Can you work these out from the model? Positions are in its coordinate system, mm. A direction names the side the tool comes from. Give positions to 0.01 mm unless a question says otherwise; leave off trailing zeros. Write each loop counter-clockwise with the first axis right and the second up, starting at its lowest first coordinate (ties: lowest second). Pieces come first, ordered by that corner, then holes.
from build123d import *

# Parameters (mm, degrees)
SKETCH1_W           = 8.6
SKETCH1_H           = 27
BOSS_EXTRUDE1_DEPTH = 31.5
SKETCH2_W           = 27
SKETCH2_H           = 3
BOSS_EXTRUDE2_DEPTH = 40.5
SKETCH3_W           = 3
SKETCH3_H           = 28.5
BOSS_EXTRUDE3_DEPTH = 40.5
SKETCH4_W           = 8.6
SKETCH4_H           = 27
BOSS_EXTRUDE4_DEPTH = 31.5
CUT_EXTRUDE8_DEPTH  = 10
FILLET1_R           = 3
SKETCH5_R           = 2.2
CUT_EXTRUDE1_DEPTH  = 5
SKETCH6_W           = 17.5
SKETCH6_H           = 10
CUT_EXTRUDE2_DEPTH  = 10
FILLET3_R           = 1
SKETCH9_W           = 27
SKETCH9_H           = 5
BOSS_EXTRUDE5_DEPTH = 22.5
SKETCH10_R          = 2.2
CUT_EXTRUDE5_DEPTH  = 100
FILLET4_R           = 3
FILLET5_R           = 0.3
SKETCH12_W          = 14.05
SKETCH12_H          = 27
CUT_EXTRUDE6_DEPTH  = 10
FILLET6_R           = 3


with BuildPart() as part:
    # Sketch1 → Boss-Extrude1 (new body)
    with BuildSketch(Plane(origin=(0, 0, 0), x_dir=(1, 0, 0), z_dir=(0, 1, 0))):
        with Locations((4.3, 0)):
            Rectangle(SKETCH1_W, SKETCH1_H)
    extrude(amount=BOSS_EXTRUDE1_DEPTH)

    # Sketch2 → Boss-Extrude2 (add)
    with BuildSketch(Plane(origin=(8.6, 0, 0), x_dir=(0, 0, -1), z_dir=(1, 0, 0))):
        with Locations((0, 1.5)):
            Rectangle(SKETCH2_W, SKETCH2_H)
    extrude(amount=BOSS_EXTRUDE2_DEPTH)

    # Sketch3 → Boss-Extrude3 (add)
    with BuildSketch(Plane(origin=(8.6, 0, 0), x_dir=(0, 0, -1), z_dir=(1, 0, 0))):
        with Locations((12, 17.25)):
            Rectangle(SKETCH3_W, SKETCH3_H)
    extrude(amount=BOSS_EXTRUDE3_DEPTH)

    # Sketch4 → Boss-Extrude4 (add)
    with BuildSketch(Plane(origin=(0, 31.5, 0), x_dir=(1, 0, 0), z_dir=(0, 1, 0))):
        with Locations((53.4, 0)):
            Rectangle(SKETCH4_W, SKETCH4_H)
    extrude(amount=-BOSS_EXTRUDE4_DEPTH)

    # Sketch15 → Cut-Extrude8 (cut)
    with BuildSketch(Plane.XY.offset(-10.5)):
        with BuildLine():
            Line((31.35, 8.25), (31.35, 26.25))
            ThreePointArc((31.35, 26.25), (28.85, 28.75), (26.35, 26.25))
            Line((26.35, 26.25), (26.35, 8.25))
            ThreePointArc((26.35, 8.25), (28.85, 5.75), (31.35, 8.25))
        make_face()
        with BuildLine():
            Line((42.725, 8.25), (42.725, 26.25))
            ThreePointArc((42.725, 26.25), (40.225, 28.75), (37.725, 26.25))
            Line((37.725, 26.25), (37.725, 8.25))
            ThreePointArc((37.725, 8.25), (40.225, 5.75), (42.725, 8.25))
        make_face()
        with BuildLine():
            Line((19.975, 8.25), (19.975, 26.25))
            ThreePointArc((19.975, 26.25), (17.475, 28.75), (14.975, 26.25))
            Line((14.975, 26.25), (14.975, 8.25))
            ThreePointArc((14.975, 8.25), (17.475, 5.75), (19.975, 8.25))
        make_face()
    extrude(amount=-CUT_EXTRUDE8_DEPTH, mode=Mode.SUBTRACT)

    # Fillet1
    fillet1_edges = [part.edges().sort_by_distance(p)[0] for p in [
        (57.7, 15.75, -13.5),
        (57.7, 15.75, 13.5),
        (49.1, 17.25, 13.5),
        (8.6, 17.25, 13.5),
    ]]
    fillet(fillet1_edges, radius=FILLET1_R)

    # Sketch5 → Cut-Extrude1 (cut)
    with BuildSketch(Plane(origin=(0, 31.5, 0), x_dir=(1, 0, 0), z_dir=(0, 1, 0))):
        with Locations(Location((53.4, 4.95, 0), (0, 0, 270))):
            Circle(SKETCH5_R)
        with Locations(Location((53.4, -4.95, 0), (0, 0, 270))):
            Circle(SKETCH5_R)
        with Locations(Location((4.3, 4.95, 0), (0, 0, 270))):
            Circle(SKETCH5_R)
        with Locations(Location((4.3, -4.95, 0), (0, 0, 270))):
            Circle(SKETCH5_R)
    extrude(amount=-CUT_EXTRUDE1_DEPTH, mode=Mode.SUBTRACT)

    # Sketch6 → Cut-Extrude2 (cut)
    with BuildSketch(Plane.ZY.offset(-49.1)):
        with Locations((4.75, 10)):
            Rectangle(SKETCH6_W, SKETCH6_H)
    extrude(amount=-CUT_EXTRUDE2_DEPTH, mode=Mode.SUBTRACT)

    # Fillet3
    fillet3_edges = [part.edges().sort_by_distance(p)[0] for p in [
        (56.821320344, 5, 12.621320344),
        (56.821320344, 15, 12.621320344),
        (57.7, 10, -4),
        (49.1, 5, 3.25),
        (49.1, 15, 3.25),
        (49.1, 10, -4),
        (49.978679656, 15, 12.621320344),
        (57.7, 15, 3.25),
        (53.4, 15, 13.5),
        (49.978679656, 5, 12.621320344),
        (57.7, 5, 3.25),
        (53.4, 15, -4),
        (53.4, 5, 13.5),
        (53.4, 5, -4),
    ]]
    fillet(fillet3_edges, radius=FILLET3_R)

    # Sketch9 → Boss-Extrude5 (add)
    with BuildSketch(Plane.ZY):
        with Locations((0, 29)):
            Rectangle(SKETCH9_W, SKETCH9_H)
        with Locations((0, 2.5)):
            Rectangle(SKETCH9_W, SKETCH9_H)
    extrude(amount=BOSS_EXTRUDE5_DEPTH)

    # Sketch10 → Cut-Extrude5 (cut)
    with BuildSketch(Plane(origin=(0, 31.5, 0), x_dir=(1, 0, 0), z_dir=(0, 1, 0))):
        with Locations(Location((-5.3, 4.95, 0), (0, 0, 90))):
            Circle(SKETCH10_R)
        with Locations(Location((-5.3, -4.95, 0), (0, 0, 90))):
            Circle(SKETCH10_R)
        with Locations(Location((-17.2, -4.95, 0), (0, 0, 90))):
            Circle(SKETCH10_R)
        with Locations(Location((-17.2, 4.95, 0), (0, 0, 90))):
            Circle(SKETCH10_R)
    extrude(amount=-CUT_EXTRUDE5_DEPTH, mode=Mode.SUBTRACT)

    # Fillet4
    fillet4_edges = [part.edges().sort_by_distance(p)[0] for p in [
        (0, 15.75, 13.5),
        (0, 15.75, -13.5),
        (-22.5, 2.5, 13.5),
        (-22.5, 2.5, -13.5),
    ]]
    fillet(fillet4_edges, radius=FILLET4_R)

    # Fillet5
    # the kernel refuses this fillet: 0.3 mm, written as the material it adds along each edge
    with BuildSketch(Plane(origin=(0, 5, 10.5), x_dir=(0, 1, 0), z_dir=(0, 0, -1))) as fillet5_piece_1:
        with BuildLine():
            CenterArc((FILLET5_R, -FILLET5_R), FILLET5_R, 90, 90)
            Line((0, -FILLET5_R), (0, 0))
            Line((0, 0), (FILLET5_R, 0))
        make_face()
    extrude(amount=21)
    with BuildSketch(Plane(origin=(0, 26.5, 10.5), x_dir=(0, -1, 0), z_dir=(0, 0, -1))) as fillet5_piece_2:
        with BuildLine():
            CenterArc((FILLET5_R, FILLET5_R), FILLET5_R, 180, 90)
            Line((0, FILLET5_R), (0, 0))
            Line((0, 0), (FILLET5_R, 0))
        make_face()
    extrude(amount=21)
    with BuildSketch(Plane(origin=(3, 5, -10.5), x_dir=(-1, 0, 0), z_dir=(0, 0, 1))) as fillet5_piece_3_section:
        with BuildLine():
            CenterArc((3 + FILLET5_R, -FILLET5_R), FILLET5_R, 90, 90)
            Line((3 + FILLET5_R, 0), (3, 0))
            Line((3, 0), (3, -FILLET5_R))
        make_face()
    fillet5_piece_3 = revolve(axis=Axis((3, 5, -10.5), (0, -1, 0)), revolution_arc=104.329698924, mode=Mode.PRIVATE)
    fillet5_piece_3 = split(fillet5_piece_3, bisect_by=Plane(origin=(0.81861369, 5.084946104, -13.5), z_dir=(0, 0, 1)), keep=Keep.TOP, mode=Mode.PRIVATE)
    add(fillet5_piece_3)
    with BuildSketch(Plane(origin=(3, 26.5, -10.5), x_dir=(-1, 0, 0), z_dir=(0, 0, 1))) as fillet5_piece_4_section:
        with BuildLine():
            CenterArc((3 + FILLET5_R, FILLET5_R), FILLET5_R, 180, 90)
            Line((3 + FILLET5_R, 0), (3, 0))
            Line((3, 0), (3, FILLET5_R))
        make_face()
    fillet5_piece_4 = revolve(axis=Axis((3, 26.5, -10.5), (0, -1, 0)), revolution_arc=104.329698924, mode=Mode.PRIVATE)
    fillet5_piece_4 = split(fillet5_piece_4, bisect_by=Plane(origin=(0.81861369, 26.415053896, -13.5), z_dir=(0, 0, 1)), keep=Keep.TOP, mode=Mode.PRIVATE)
    add(fillet5_piece_4)
    with BuildSketch(Plane(origin=(3, 5, 10.5), x_dir=(0.24750126301206385, 0, 0.968887570777659), z_dir=(0.968887570777659, 0, -0.24750126301206385))) as fillet5_piece_5_section:
        with BuildLine():
            CenterArc((3 + FILLET5_R, -FILLET5_R), FILLET5_R, 90, 90)
            Line((3 + FILLET5_R, 0), (3, 0))
            Line((3, 0), (3, -FILLET5_R))
        make_face()
    fillet5_piece_5 = revolve(axis=Axis((3, 5, 10.5), (0, -1, 0)), revolution_arc=104.329698924, mode=Mode.PRIVATE)
    fillet5_piece_5 = split(fillet5_piece_5, bisect_by=Plane(origin=(0.818613701, 5.084946089, 13.5), z_dir=(0, 0, -1)), keep=Keep.TOP, mode=Mode.PRIVATE)
    add(fillet5_piece_5)
    with BuildSketch(Plane(origin=(3, 26.5, 10.5), x_dir=(0.24750126301206454, 0, 0.9688875707776589), z_dir=(0.9688875707776589, 0, -0.24750126301206454))) as fillet5_piece_6_section:
        with BuildLine():
            CenterArc((3 + FILLET5_R, FILLET5_R), FILLET5_R, 180, 90)
            Line((3, FILLET5_R), (3, 0))
            Line((3, 0), (3 + FILLET5_R, 0))
        make_face()
    fillet5_piece_6 = revolve(axis=Axis((3, 26.5, 10.5), (0, -1, 0)), revolution_arc=104.329698924, mode=Mode.PRIVATE)
    fillet5_piece_6 = split(fillet5_piece_6, bisect_by=Plane(origin=(0.818613746, 26.41505391, 13.5), z_dir=(0, 0, -1)), keep=Keep.TOP, mode=Mode.PRIVATE)
    add(fillet5_piece_6)

    # Sketch12 → Cut-Extrude6 (cut)
    with BuildSketch(Plane(origin=(0, 31.5, 0), x_dir=(1, 0, 0), z_dir=(0, 1, 0))):
        with Locations((-15.475, 0)):
            Rectangle(SKETCH12_W, SKETCH12_H)
    extrude(amount=-CUT_EXTRUDE6_DEPTH, mode=Mode.SUBTRACT)

    # Fillet6
    fillet6_edges = [part.edges().sort_by_distance(p)[0] for p in [
        (-8.45, 29, -13.5),
        (-8.45, 29, 13.5),
    ]]
    fillet(fillet6_edges, radius=FILLET6_R)


solid = part.part
(1) If I drill on L1, parallel to Z at x = -17.2, y = 2.65; L2, parallel to X at y = 29.8, z = -4.95; L3, parallel to X at y = 1.75, z = 4.95, over which ranges is the centre line in solid material (lowest first)?
Returned:
L1: z = -13.5 to -7.15, -2.75 to 2.75, 7.15 to 13.5
L2: x = -8.45 to -7.5, -3.1 to 2.1, 6.5 to 8.6, 49.1 to 51.2, 55.6 to 57.7
L3: x = -22.5 to -19.4, -15 to -7.5, -3.1 to 57.7
(2) Imagine slicing it at D-D, the plane x = 4.3. Write out the boundary of the cut face in (y, z).
Returned:
outline: (0, -13.5) - (31.5, -13.5) - (31.5, -7.15) - (26.5, -7.15) - (26.5, -2.75) - (31.5, -2.75) - (31.5, 2.75) - (26.5, 2.75) - (26.5, 7.15) - (31.5, 7.15) - (31.5, 13.5) - (0, 13.5) - close
(3) Imagine slicing it at C-C, the plane x = -17.2. Write out the boundary of the cut face in (y, z).
Returned:
outline: (0, -13.5) - (5, -13.5) - (5, -7.15) - (0, -7.15) - close; (0, -2.75) - (5, -2.75) - (5, 2.75) - (0, 2.75) - close; (0, 7.15) - (5, 7.15) - (5, 13.5) - (0, 13.5) - close
(4) Imagine slicing it at A-A, the plane z = -1.75. Write out the boundary of the cut face in (x, y).
Returned:
outline: (-22.5, 0) - (57.7, 0) - (57.7, 4) arc R1 ccw to (56.7, 5) - (50.1, 5) arc R1 ccw to (49.1, 4) - (49.1, 3) - (8.6, 3) - (8.6, 31.5) - (-8.45, 31.5) - (-8.45, 26.5) - (-0.3, 26.5) arc R0.3 cw to (0, 26.2) - (0, 5.3) arc R0.3 cw to (-0.3, 5) - (-22.5, 5) - close; (49.1, 16) arc R1 ccw to (50.1, 15) - (56.7, 15) arc R1 ccw to (57.7, 16) - (57.7, 31.5) - (49.1, 31.5) - close
(5) Will these pins go through, and if not, where does the flat tip stop? P1, Ø0.9, axis at y = 17.5, z = -12.5, coming from the +X side; P2, Ø1, axis at x = 4, z = 5, coming from the +Y side; P3, Ø5.5, axis at x = 52.5, y = 12, coming from the +Z side.
Returned:
P1: stops at x = 57.27
P2: stops at y = 26.5
P3: stops at z = -3.66
(6) If we mould it in two halves opening along Z, with no side actions, what happens to faces 1 (the face through (0.86, 15.9, 12.6)), 2 (the face through (4, 26.5, 5)), 3 (the face through (49.1, 21, -2)), 4 (the face through (5.79, 29.04, -6.57))? For each: +Z half, -Z half, draft (parallel to the pull), parting line (faces both ways), or undercut.
Returned:
face 1: +Z half
face 2: undercut
face 3: draft
face 4: undercut
(7) Imagine slicing it at B-B, the plane y = 22.5. Write out the boundary of the cut face in (x, z) (3 decimals), plus the area to 3 significant figures.
Returned:
outline: (0, -10.5) arc R3 ccw to (3, -13.5) - (14.975, -13.5) - (14.975, -10.5) - (8.6, -10.5) - (8.6, 10.5) arc R3 ccw to (5.6, 13.5) - (3, 13.5) arc R3 ccw to (0, 10.5) - close; (19.975, -13.5) - (26.35, -13.5) - (26.35, -10.5) - (19.975, -10.5) - close; (31.35, -13.5) - (37.725, -13.5) - (37.725, -10.5) - (31.35, -10.5) - close; (42.725, -13.5) - (54.7, -13.5) arc R3 ccw to (57.7, -10.5) - (57.7, 10.5) arc R3 ccw to (54.7, 13.5) - (52.1, 13.5) arc R3 ccw to (49.1, 10.5) - (49.1, -10.5) - (42.725, -10.5) - close
area: 529 mm2
(8) For faces 5 (the face through (0.9, 15.9, -12.64)), 6 (the face through (53, 26.5, -5)), 7 (the face through (31.35, 17, -12)), 8 (the face through (-6.79, 29.04, 6.57)), 9 (the face through (29, 3, 2)), which set-ups out of +Z, -Z, +X, -X, +Y, -Y let a thin tool reach every point of the face, with its end or its side?
Returned:
face 5: -Z, -X
face 6: +Y
face 7: +Z, -Z
face 8: +Y, -Y
face 9: +Z, +Y
